from build123d import *

# Parameters (mm, degrees)
SKETCH5_R           = 73.025
SKETCH5_R_2         = 3.175
PLATEBASE_DEPTH     = 6.35
PLATETOP_DEPTH      = 9.525
SKETCH9_R           = 73.025
SKETCH9_R_2         = 66.675
PLATEWALLS_DEPTH    = 9.525
PLATESLOTENDS_DEPTH = 9.525
BATTERYSLOT_DEPTH   = 9.525
SKETCH13_R          = 4.765
INSERTHOLE_DEPTH    = 8.128
INSERTHOLES_COUNT   = 4


with BuildPart() as part:
    # Sketch5 → PlateBase (new body)
    with BuildSketch(Plane(origin=(0, 0, 0), x_dir=(1, 0, 0), z_dir=(0, 1, 0))):
        Circle(SKETCH5_R)
        with Locations((38.1, 38.1)):
            Circle(SKETCH5_R_2, mode=Mode.SUBTRACT)
        with Locations((38.1, -38.1)):
            Circle(SKETCH5_R_2, mode=Mode.SUBTRACT)
        with Locations((-38.1, 38.1)):
            Circle(SKETCH5_R_2, mode=Mode.SUBTRACT)
        with Locations((-38.1, -38.1)):
            Circle(SKETCH5_R_2, mode=Mode.SUBTRACT)
    extrude(amount=PLATEBASE_DEPTH)

    # Sketch6 → PlateTop (add)
    with BuildSketch(Plane(origin=(0, 6.35, 0), x_dir=(1, 0, 0), z_dir=(0, 1, 0))):
        with BuildLine():
            Line((-3.175, 0), (-3.175, 72.955945611))
            ThreePointArc((-3.175, 72.955945611), (-6.35605636, 72.747860261), (-9.525, 72.401139494))
            Line((-9.525, 72.401139494), (-9.525, 0))
            Line((-9.525, 0), (-9.525, -72.401139494))
            ThreePointArc((-9.525, -72.401139494), (-6.35605636, -72.747860261), (-3.175, -72.955945611))
            Line((-3.175, -72.955945611), (-3.175, 0))
        make_face()
        with BuildLine():
            Line((3.175, 72.955945611), (3.175, 0))
            Line((3.175, 0), (3.175, -72.955945611))
            ThreePointArc((3.175, -72.955945611), (6.35605636, -72.747860261), (9.525, -72.401139494))
            Line((9.525, -72.401139494), (9.525, 0))
            Line((9.525, 0), (9.525, 72.401139494))
            ThreePointArc((9.525, 72.401139494), (6.35605636, 72.747860261), (3.175, 72.955945611))
        make_face()
    extrude(amount=PLATETOP_DEPTH)

    # Sketch9 → PlateWalls (add)
    with BuildSketch(Plane(origin=(0, 6.35, 0), x_dir=(1, 0, 0), z_dir=(0, 1, 0))):
        Circle(SKETCH9_R)
        Circle(SKETCH9_R_2, mode=Mode.SUBTRACT)
    extrude(amount=PLATEWALLS_DEPTH)

    # Sketch11 → PlateSlotEnds (add)
    with BuildSketch(Plane(origin=(0, 6.35, 0), x_dir=(1, 0, 0), z_dir=(0, 1, 0))):
        with BuildLine():
            Line((-3.175, -63.5), (3.175, -63.5))
            Line((3.175, -63.5), (3.175, -66.599361859))
            ThreePointArc((3.175, -66.599361859), (0, -66.675), (-3.175, -66.599361859))
            Line((-3.175, -66.599361859), (-3.175, -63.5))
        make_face()
        with BuildLine():
            Line((-3.175, 63.5), (3.175, 63.5))
            Line((3.175, 63.5), (3.175, 66.599361859))
            ThreePointArc((3.175, 66.599361859), (0, 66.675), (-3.175, 66.599361859))
            Line((-3.175, 66.599361859), (-3.175, 63.5))
        make_face()
    extrude(amount=PLATESLOTENDS_DEPTH)

    # Sketch12 → BatterySlot (add)
    with BuildSketch(Plane(origin=(0, 6.35, 0), x_dir=(1, 0, 0), z_dir=(0, 1, 0))):
        with BuildLine():
            Line((-9.525, -65.991135768), (-9.525, -56.958062669))
            Line((-9.525, -56.958062669), (-25.527, -56.958062669))
            Line((-25.527, -56.958062669), (-25.527, -26.986062669))
            Line((-25.527, -26.986062669), (-9.525, -26.986062669))
            Line((-9.525, -26.986062669), (-9.525, -21.948739215))
            Line((-9.525, -21.948739215), (-30.607, -21.948739215))
            Line((-30.607, -21.948739215), (-30.607, -59.234847649))
            ThreePointArc((-30.607, -59.234847649), (-20.348371269, -63.494089581), (-9.525, -65.991135768))
        make_face()
    extrude(amount=BATTERYSLOT_DEPTH)

    # Sketch13 → InsertHole (cut)
    with BuildSketch(Plane.XY.offset(73.025)):
        with Locations((0, 7.9375)):
            Circle(SKETCH13_R)
    inserthole = extrude(amount=-INSERTHOLE_DEPTH, mode=Mode.SUBTRACT)

    # InsertHoles: InsertHole ×4 about axis
    insertholes_axis = Axis((0, 0, 0), (0, 1, 0))
    for i in range(1, INSERTHOLES_COUNT):
        add(inserthole.rotate(insertholes_axis, i * 360 / INSERTHOLES_COUNT), mode=Mode.SUBTRACT)


solid = part.part
Verification items for the finished model (mm, model axes). A direction names the side the tool comes from. Give positions to 0.01 mm unless a question says otherwise; leave off trailing zeros. Write each loop counter-clockwise with the first axis right and the second up, starting at its lowest first coordinate (ties: lowest second). Pieces come first, ordered by that corner, then holes.
(1) Gauge pin test, flat ends, axial feed: pin 1 (2 mm diameter, centred on y = 6.5, z = -20.5, fed in from -X); pin 2 (8 mm diameter, centred on y = 13, z = 47, fed in from +X); pin 3 (5 mm diameter, centred on y = 12, z = 48, fed in from -X); pin 4 (17.5 mm diameter, centred on x = -16.5, z = 36.5, fed in from +Y) (3 decimals). Record the tip position at first contact, or that the pin passes through.
(2) Cross-section at A-A (z = 0). State how many separate pieces and enclosed holes the cut face has, plus the area to 3 significant figures.
(3) Material ranges on line 1 (Y direction, x = 68, z = 0) (1 decimal); line 2 (X direction, y = 9.25, z = 57) (3 decimals); line 3 (X direction, y = 3.5, z = -38.1) (3 decimals), recorded low to high.
(4) Access from +Z, -Z, +X, -X, +Y, -Y to the whole of each face (thin tool, end or side, straight path). Record for faces 1 (the face through (-9.525, 11, 42)), 2 (the face through (0.62, 12.66, -69.02)), 3 (the face through (0, 8, 64.897)).
(5) Cross-section at D-D (z = -38.1). Enter the section's corners in (x, y) (3 decimals), plus the area to 3 significant figures.
(6) Cross-section at B-B (x = 38.1). Enter the section's corners in (y, z) (3 decimals).
(7) Mould release check, pull along X, two halves, no side actions. Record for faces 4 (the face through (-69.02, 3.71, 2.2)), 5 (the face through (0, 6.35, -1)), 6 (the face through (31, 6.35, -1)), 7 (the face through (64.897, 5, 0)): +X half, -X half, draft (parallel to the pull), parting line (faces both ways), or undercut.
Worked out:
1. pin 1: stops at x = -70.37
1. pin 2: stops at x = 59.02
1. pin 3: stops at x = -57.12
1. pin 4: stops at y = 15.875
2. separate pieces: 3
2. enclosed holes: 0
2. area: 1,040 mm2
3. line 1: y = 0 to 3.2, 12.7 to 15.9
3. line 2: x = -45.647 to -34.591, -30.607 to -3.175, 3.175 to 9.525, 34.591 to 45.647
3. line 3: x = -62.298 to -41.275, -34.925 to 34.925, 41.275 to 62.298
4. face 1: +Y
4. face 2: -Z
4. face 3: +Z
5. outline: (-62.298, 0) - (-41.275, 0) - (-41.275, 6.35) - (-54.717, 6.35) - (-54.717, 15.875) - (-62.298, 15.875) - close; (-34.925, 0) - (34.925, 0) - (34.925, 6.35) - (9.525, 6.35) - (9.525, 15.875) - (3.175, 15.875) - (3.175, 6.35) - (-3.175, 6.35) - (-3.175, 15.875) - (-9.525, 15.875) - (-9.525, 6.35) - (-34.925, 6.35) - close; (41.275, 0) - (62.298, 0) - (62.298, 15.875) - (54.717, 15.875) - (54.717, 6.35) - (41.275, 6.35) - close
5. area: 976 mm2
6. outline: (0, -62.298) - (15.875, -62.298) - (15.875, -54.717) - (6.35, -54.717) - (6.35, -41.275) - (0, -41.275) - close; (0, -34.925) - (6.35, -34.925) - (6.35, 34.925) - (0, 34.925) - close; (0, 41.275) - (6.35, 41.275) - (6.35, 54.717) - (15.875, 54.717) - (15.875, 62.298) - (0, 62.298) - close
7. face 4: draft
7. face 5: undercut
7. face 6: undercut
7. face 7: +X half
